Verification items for the finished model (mm, model axes). Face numbers are marked on the shaded views. A direction names the side the tool comes from. Round coordinates to 2 decimals unless told otherwise and drop trailing zeros. Write each loop counter-clockwise with the first axis right and the second up, starting at its lowest first coordinate (ties: lowest second). Pieces come first, ordered by that corner, then holes.
from build123d import *

# Parameters (mm, degrees)
F0_W      = 16
F0_H      = 8
F1_DEPTH  = 10.5
F2_R      = 0.875
F3_DEPTH  = 0.5
F4_W      = 16
F4_H      = 8
F5_DEPTH  = 3.5
F7_DEPTH  = 25
F9_DEPTH  = 2
F10_DEPTH = 25
F11_DEPTH = 25
F12_DEPTH = 25
F13_R     = 2
F13_R_2   = 0.5
F14_DEPTH = 3


with BuildPart() as f1:
    # F0 (on Top) → F1 (new body)
    with BuildSketch(Plane.XY):
        Rectangle(F0_W, F0_H)
    extrude(amount=F1_DEPTH)

    # F2 (on face) → F3 (join)
    with BuildSketch(Plane.XY.offset(10.5)):
        with BuildLine():
            ThreePointArc((9.75, -4), (11.25, 0), (9.75, 4))
            Line((9.75, 4), (-9.75, 4))
            ThreePointArc((-9.75, 4), (-11.25, 0), (-9.75, -4))
            Line((-9.75, -4), (9.75, -4))
        make_face()
        with Locations((-9.5, 0)):
            Circle(F2_R, mode=Mode.SUBTRACT)
        with Locations((9.5, 0)):
            Circle(F2_R, mode=Mode.SUBTRACT)
    extrude(amount=F3_DEPTH)

    # F4 (on face) → F5 (join)
    with BuildSketch(Plane.XY.offset(11)):
        Rectangle(F4_W, F4_H)
    extrude(amount=F5_DEPTH)

    # F6 (on face) → F7 (cut)
    with BuildSketch(Plane.XZ.offset(4)):
        Polygon((-8, 14.5), (-8, 13), (-4, 14.5), align=None)
    extrude(amount=-F7_DEPTH, mode=Mode.SUBTRACT)

    # F8 (on face) → F9 (join)
    with BuildSketch(Plane.XY.offset(14.5)):
        with BuildLine():
            ThreePointArc((0.4292361111, -1.9110586725), (4.9851157927, -3.928364402), (8.05, 0))
            ThreePointArc((8.05, 0), (4.9851157927, 3.928364402), (0.4292361111, 1.9110586725))
            ThreePointArc((0.4292361111, 1.9110586725), (1.3014232895, 1.1271641992), (1.625, 0))
            ThreePointArc((1.625, 0), (1.3014232895, -1.1271641992), (0.4292361111, -1.9110586725))
        make_face()
        with BuildLine():
            ThreePointArc((1.625, 0), (1.3014232895, 1.1271641992), (0.4292361111, 1.9110586725))
            ThreePointArc((0.4292361111, 1.9110586725), (-0.05, 0), (0.4292361111, -1.9110586725))
            ThreePointArc((0.4292361111, -1.9110586725), (1.3014232895, -1.1271641992), (1.625, 0))
        make_face()
        with BuildLine():
            ThreePointArc((0.4292361111, -1.9110586725), (-0.05, 0), (0.4292361111, 1.9110586725))
            ThreePointArc((0.4292361111, 1.9110586725), (-2.625, 0), (0.4292361111, -1.9110586725))
        make_face()
    extrude(amount=F9_DEPTH)

    # F10 (cut): a face of the model
    f10_faces = [f1.faces().sort_by_distance(p)[0] for p in [
        (4, 4.0200106199, 14.5),
    ]]
    extrude(f10_faces, amount=-F10_DEPTH, mode=Mode.SUBTRACT)

    # F11 (cut): a face of the model
    f11_faces = [f1.faces().sort_by_distance(p)[0] for p in [
        (4, -4.0200106199, 14.5),
    ]]
    extrude(f11_faces, amount=-F11_DEPTH, mode=Mode.SUBTRACT)

    # F12 (cut): a face of the model
    f12_faces = [f1.faces().sort_by_distance(p)[0] for p in [
        (8.0200106199, 0, 14.5),
    ]]
    extrude(f12_faces, amount=-F12_DEPTH, mode=Mode.SUBTRACT)

    # F13 (on face) → F14 (join)
    with BuildSketch(Plane.XY.offset(16.5)):
        with Locations((4, 0)):
            Circle(F13_R)
        with Locations((4, 0)):
            Circle(F13_R_2, mode=Mode.SUBTRACT)
    extrude(amount=F14_DEPTH)


solid = f1.part
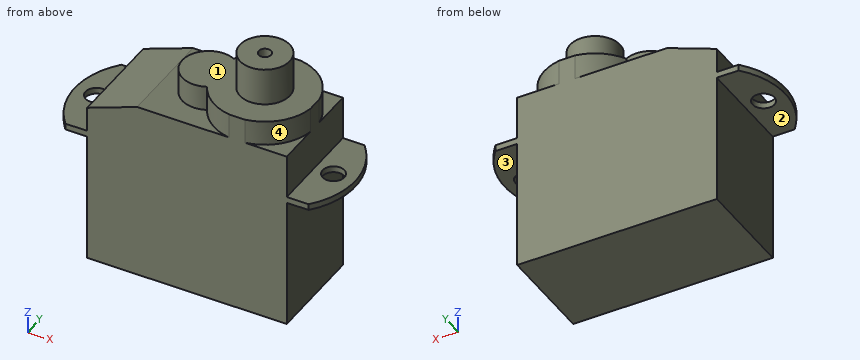
Q1. Material ranges on line 1 along Y through (x, z) = (4, 17.2); line 2 along Z through (x, y) = (6.5, 0.75); line 3 along X through (y, z) = (-2.75, 11.5), recorded low to high.
Recorded:
line 1: y = -2 to -0.5, 0.5 to 2
line 2: z = 0 to 16.5
line 3: x = -8 to 8
Q2. Sectioned sample at D-D (x = 4). Enter the section's corners in (y, z).
Recorded:
outline: (-4, 0) - (4, 0) - (4, 16.5) - (2, 16.5) - (2, 19.5) - (0.5, 19.5) - (0.5, 16.5) - (-0.5, 16.5) - (-0.5, 19.5) - (-2, 19.5) - (-2, 16.5) - (-4, 16.5) - close
Q3. Sectioned sample at A-A (x = -9.5). Enter the section's corners in (y, z) (3 decimals).
Recorded:
outline: (-4, 10.5) - (-0.875, 10.5) - (-0.875, 11) - (-4, 11) - close; (0.875, 10.5) - (4, 10.5) - (4, 11) - (0.875, 11) - close
Q4. Sectioned sample at B-B (y = 0). Give the number of separate pieces and of enclosed holes in the cut face, plus the area to 3 significant figures.
Recorded:
separate pieces: 3
enclosed holes: 0
area: 261 mm2
Q5. Tool access check on the marked faces 1, 2, 3 and 4. Record the directions out of +Z, -Z, +X, -X, +Y, -Y that give a thin tool (end or side, any length) a straight path to the whole face; none if there is none.
Recorded:
face 1: +Z
face 2: -Z, -X, +Y, -Y
face 3: -Z, +X, +Y, -Y
face 4: +Z, +X, -Y
Q6. Depth check by flat-ended pin: P1, Ø0.6, axis at y = 2, z = 12.5, coming from the -X side; P2, Ø2, axis at x = -1.5, y = 1, coming from the +Z side; P3, Ø3.5, axis at x = -9.5, y = -1.5, coming from the +Z side. Enter the tip coordinate at first touch or a pass-through.
Recorded:
P1: stops at x = -8
P2: stops at z = 16.5
P3: stops at z = 13.09
Q7. Sectioned sample at C-C (z = 15.5). Enter the section's corners in (x, y) (3 decimals), plus the area to 3 significant figures.
Recorded:
outline: (0.429, -1.911) arc R4.05 ccw to (3.366, -4) - (4.634, -4) arc R4.05 ccw to (8, -0.634) - (8, 0.634) arc R4.05 ccw to (4.634, 4) - (3.366, 4) arc R4.05 ccw to (0.429, 1.911) arc R2.125 ccw (long way) to start
area: 61.1 mm2
